from build123d import *

# Parameters (mm, degrees)
BOSS_EXTRUDE3_DEPTH        = 7.1501
SKETCH5_R                  = 4.826
CUT_EXTRUDE4_DEPTH         = 33.306330486
SKETCH6_R                  = 14.2875
CUT_EXTRUDE5_DEPTH         = 3.2131
TAP_DRILL_FOR_3_48_TAP2_D  = 1.9939
TAP_DRILL_FOR_10_32_TAP3_D = 4.0386
FILLET3_R                  = 0.508
FILLET4_R                  = 0.508
FILLET5_R                  = 0.508
FILLET6_R                  = 0.508


with BuildPart() as part:
    # Sketch1 → Boss-Extrude3 (new body)
    with BuildSketch(Plane(origin=(0, 0, 0), x_dir=(0, 0, -1), z_dir=(1, 0, 0))):
        with BuildLine():
            Line((9.216458059, 14.457106413), (23.495, 5.354483857))
            ThreePointArc((23.495, 5.354483857), (26.431497015, 0), (23.495, -5.354483857))
            Line((23.495, -5.354483857), (9.216458059, -14.457106413))
            ThreePointArc((9.216458059, -14.457106413), (0, -17.145), (-9.216458059, -14.457106413))
            Line((-9.216458059, -14.457106413), (-23.495, -5.354483857))
            ThreePointArc((-23.495, -5.354483857), (-26.431497015, 0), (-23.495, 5.354483857))
            Line((-23.495, 5.354483857), (-9.216458059, 14.457106413))
            ThreePointArc((-9.216458059, 14.457106413), (0, 17.145), (9.216458059, 14.457106413))
        make_face()
    extrude(amount=BOSS_EXTRUDE3_DEPTH)

    # Sketch5 → Cut-Extrude4 (cut, through all)
    with BuildSketch(Plane(origin=(7.1501, 0, 0), x_dir=(0, 0, -1), z_dir=(1, 0, 0))):
        Circle(SKETCH5_R)
    extrude(amount=-CUT_EXTRUDE4_DEPTH, mode=Mode.SUBTRACT)

    # Sketch6 → Cut-Extrude5 (cut)
    with BuildSketch(Plane(origin=(7.1501, 0, 0), x_dir=(0, 0, -1), z_dir=(1, 0, 0))):
        Circle(SKETCH6_R)
    extrude(amount=-CUT_EXTRUDE5_DEPTH, mode=Mode.SUBTRACT)

    # Tap Drill for #3-48 Tap2 (through all)
    with Locations(Plane(origin=(3.937, 0, 0), x_dir=(0, 0, -1), z_dir=(1, 0, 0))):
        with Locations((0, 7.4422), (0, -7.4422), (6.44513426, 3.7211), (-6.44513426, -3.7211)):
            Hole(TAP_DRILL_FOR_3_48_TAP2_D / 2)

    # Tap Drill for #10-32 Tap3 (through all)
    with Locations(Plane(origin=(7.1501, 0, 0), x_dir=(0, 0, -1), z_dir=(1, 0, 0))):
        with Locations((-22.86, 0), (22.86, 0)):
            Hole(TAP_DRILL_FOR_10_32_TAP3_D / 2)

    # Fillet3
    fillet3_edges = [part.edges().sort_by_distance(p)[0] for p in [
        (7.1501, 0, 14.2875),
    ]]
    fillet(fillet3_edges, radius=FILLET3_R)

    # Fillet4
    fillet4_edges = [part.edges().sort_by_distance(p)[0] for p in [
        (3.937, 0, 4.826),
    ]]
    fillet(fillet4_edges, radius=FILLET4_R)

    # Fillet5
    fillet5_edges = [part.edges().sort_by_distance(p)[0] for p in [
        (7.1501, 0, 26.431497015),
        (7.1501, -9.905795135, 16.355729029),
        (7.1501, -17.145, 0),
        (7.1501, -9.905795135, -16.355729029),
        (7.1501, 0, -26.431497015),
        (7.1501, 9.905795135, -16.355729029),
        (7.1501, 17.145, 0),
        (7.1501, 9.905795135, 16.355729029),
    ]]
    fillet(fillet5_edges, radius=FILLET5_R)

    # Fillet6
    fillet6_edges = [part.edges().sort_by_distance(p)[0] for p in [
        (0, 9.905795135, 16.355729029),
        (0, 17.145, 0),
        (0, 9.905795135, -16.355729029),
        (0, 0, -26.431497015),
        (0, -9.905795135, -16.355729029),
        (0, -17.145, 0),
        (0, -9.905795135, 16.355729029),
        (0, 0, 26.431497015),
    ]]
    fillet(fillet6_edges, radius=FILLET6_R)


solid = part.part
Design review of the part built by this model. Coordinates are the model's own, in mm. A direction names the side the tool comes from. Coordinates: 2 decimals unless noted, no trailing zeros. Order: outer loops, then holes, each group sorted by start corner. A loop starts at its lowest first (then second) coordinate and runs counter-clockwise, first axis right, second up. Notation, with made-up numbers: M 32.25,-14 L 63.25,-14 A34 ccw 63.25,19 Z; hole C 88.25,76.25 d5. An arc over 180 degrees is marked long. Use a Markdown table: item, result.
(1) Wall thickness on probe 1 along Z at (x, y) = (2, -4); probe 2 along Z at (x, y) = (1.75, -3.5); probe 3 along X at (y, z) = (9, 6): over which ranges is each line inside the solid? List them lowest first.
Worked answers:
| item | result |
|---|---|
| probe 1 | z = -25.01 to -2.7, 2.7 to 5.49, 7.4 to 25.01 |
| probe 2 | z = -25.38 to -3.32, 3.32 to 5.47, 7.42 to 25.38 |
| probe 3 | x = 0 to 3.94 |
(2) For faces 1 (the cylindrical face through (5.308, 0.628, 14.274)), 2 (the cylindrical face through (3.532, 17.144, 0.136)), list the 3-axis set-ups (+Z, -Z, +X, -X, +Y, -Y) from which the entire face can be reached by the end or side of a thin tool; tool diameter is ignored.
Worked answers:
| item | result |
|---|---|
| face 1 | +X |
| face 2 | +X, -X, +Y |
(3) Add section B-B (x = 5.5). Count the separate pieces of the cut face and the enclosed holes in it, then the cut area to 3 significant figures.
Worked answers:
| item | result |
|---|---|
| separate pieces | 1 |
| enclosed holes | 3 |
| area | 543 mm2 |
(4) Add section A-A (z = 0). Give the boundary of the cut face in (x, y) (1 decimal).
Worked answers:
| item | result |
|---|---|
| outline | M 0,-16.6 A0.5 ccw 0.5,-17.1 L 6.6,-17.1 A0.5 ccw 7.2,-16.6 L 7.2,-14.8 A0.5 ccw 6.6,-14.3 L 3.9,-14.3 L 3.9,-8.4 L 0,-8.4 Z; M 0,-6.4 L 3.9,-6.4 L 3.9,-5.3 A0.5 ccw 3.4,-4.8 L 0,-4.8 Z; M 0,4.8 L 3.4,4.8 A0.5 ccw 3.9,5.3 L 3.9,6.4 L 0,6.4 Z; M 0,8.4 L 3.9,8.4 L 3.9,14.3 L 6.6,14.3 A0.5 ccw 7.2,14.8 L 7.2,16.6 A0.5 ccw 6.6,17.1 L 0.5,17.1 A0.5 ccw 0,16.6 Z |
(5) For P1, Ø6, axis at y = -5.5, z = 17.5, coming from the -X side; P2, Ø3, axis at y = 3.72, z = -6.45, coming from the +X side; P3, Ø6, axis at y = 0, z = 0, coming from the +X side; P4, Ø2, axis at x = 1, z = 8, coming from the -Y side, all flat-tipped, find the tip position at first contact; note any pin that passes through.
Worked answers:
| item | result |
|---|---|
| P1 | stops at x = 0 |
| P2 | stops at x = 3.94 |
| P3 | passes through |
| P4 | stops at y = -15.65 |
(6) Draft analysis for pull direction Z (two halves, no side actions). For faces 3 (the cylindrical face through (3.532, -17.144, -0.136)), 4 (the flat face through (3.532, 9.97, -16.256)), 5 (the cylindrical face through (1.94, 6.47, -0.22)), state which applies: released by +Z, released by -Z, zero draft, split by the parting line, or undercut.
Worked answers:
| item | result |
|---|---|
| face 3 | split by the parting line |
| face 4 | released by -Z |
| face 5 | undercut |
